from build123d import *

# Parameters (mm, degrees)
SKETCH_1_R               = 4.95
EXTRUDE_1_DEPTH          = 4.5
CUT_EXTRUDE_1_DEPTH      = 2
PATTERN_CIRCULAR_1_COUNT = 6
MIRROR_1_COPY_1_DEPTH    = 2
MIRROR_1_COPY_2_DEPTH    = 2
MIRROR_1_COPY_3_DEPTH    = 2
MIRROR_1_COPY_4_DEPTH    = 2
MIRROR_1_COPY_5_DEPTH    = 2
EXTRUDE_2_DEPTH          = 2.4
SKETCH_5_R               = 4.95
EXTRUDE_3_DEPTH          = 22
CUT_EXTRUDE_2_DEPTH      = 29.583255588
CUT_EXTRUDE_2_DEPTH_BACK = 29.583255588
SKETCH_6_W               = 3
SKETCH_6_H               = 3


with BuildPart() as part:
    # 草图1 → 凸台-拉伸1 (new body)
    with BuildSketch(Plane.XY):
        Circle(SKETCH_1_R)
    extrude_1 = extrude(amount=EXTRUDE_1_DEPTH)

    # 草图2 → 切除-拉伸1 (cut)
    with BuildSketch(Plane(origin=(0, 0, 0), x_dir=(-1, 0, 0), z_dir=(0, 0, -1))):
        with BuildLine():
            Line((0, 4.95), (0, 3.95))
            ThreePointArc((0, 3.95), (1.022335228, 3.815407014), (1.975, 3.420800345))
            Line((1.975, 3.420800345), (2.475, 4.286825749))
            ThreePointArc((2.475, 4.286825749), (1.281154273, 4.78133284), (0, 4.95))
        make_face()
    cut_extrude_1 = extrude(amount=-CUT_EXTRUDE_1_DEPTH, mode=Mode.SUBTRACT)

    # 阵列(圆周)1: 切除-拉伸1 ×6 about axis
    pattern_circular_1_axis = Axis((0, 0, 0), (0, 0, 1))
    for i in range(1, PATTERN_CIRCULAR_1_COUNT):
        add(cut_extrude_1.rotate(pattern_circular_1_axis, i * 360 / PATTERN_CIRCULAR_1_COUNT), mode=Mode.SUBTRACT)

    # 镜向1: 凸台-拉伸1, 切除-拉伸1 across plane
    add(extrude_1.mirror(Plane.XY))
    add(cut_extrude_1.mirror(Plane.XY), mode=Mode.SUBTRACT)

    # 镜向1 copy 1 sketch → 镜向1 copy 1 (cut)
    with BuildSketch(Plane(origin=(0, 0, 0), x_dir=(-0.5000000000000001, -0.8660254037844386, 0), z_dir=(0, 0, 1))):
        with BuildLine():
            Line((0, -4.95), (0, -3.95))
            ThreePointArc((0, -3.95), (1.022335228, -3.815407014), (1.975, -3.420800345))
            Line((1.975, -3.420800345), (2.475, -4.286825749))
            ThreePointArc((2.475, -4.286825749), (1.281154273, -4.78133284), (0, -4.95))
        make_face()
    extrude(amount=-MIRROR_1_COPY_1_DEPTH, mode=Mode.SUBTRACT)

    # 镜向1 copy 2 sketch → 镜向1 copy 2 (cut)
    with BuildSketch(Plane(origin=(0, 0, 0), x_dir=(0.4999999999999998, -0.8660254037844387, 0), z_dir=(0, 0, 1))):
        with BuildLine():
            Line((0, -4.95), (0, -3.95))
            ThreePointArc((0, -3.95), (1.022335228, -3.815407014), (1.975, -3.420800345))
            Line((1.975, -3.420800345), (2.475, -4.286825749))
            ThreePointArc((2.475, -4.286825749), (1.281154273, -4.78133284), (0, -4.95))
        make_face()
    extrude(amount=-MIRROR_1_COPY_2_DEPTH, mode=Mode.SUBTRACT)

    # 镜向1 copy 3 sketch → 镜向1 copy 3 (cut)
    with BuildSketch(Plane.XY):
        with BuildLine():
            Line((0, -4.95), (0, -3.95))
            ThreePointArc((0, -3.95), (1.022335228, -3.815407014), (1.975, -3.420800345))
            Line((1.975, -3.420800345), (2.475, -4.286825749))
            ThreePointArc((2.475, -4.286825749), (1.281154273, -4.78133284), (0, -4.95))
        make_face()
    extrude(amount=-MIRROR_1_COPY_3_DEPTH, mode=Mode.SUBTRACT)

    # 镜向1 copy 4 sketch → 镜向1 copy 4 (cut)
    with BuildSketch(Plane(origin=(0, 0, 0), x_dir=(0.5000000000000004, 0.8660254037844384, 0), z_dir=(0, 0, 1))):
        with BuildLine():
            Line((0, -4.95), (0, -3.95))
            ThreePointArc((0, -3.95), (1.022335228, -3.815407014), (1.975, -3.420800345))
            Line((1.975, -3.420800345), (2.475, -4.286825749))
            ThreePointArc((2.475, -4.286825749), (1.281154273, -4.78133284), (0, -4.95))
        make_face()
    extrude(amount=-MIRROR_1_COPY_4_DEPTH, mode=Mode.SUBTRACT)

    # 镜向1 copy 5 sketch → 镜向1 copy 5 (cut)
    with BuildSketch(Plane(origin=(0, 0, 0), x_dir=(-0.5000000000000001, 0.8660254037844386, 0), z_dir=(0, 0, 1))):
        with BuildLine():
            Line((0, -4.95), (0, -3.95))
            ThreePointArc((0, -3.95), (1.022335228, -3.815407014), (1.975, -3.420800345))
            Line((1.975, -3.420800345), (2.475, -4.286825749))
            ThreePointArc((2.475, -4.286825749), (1.281154273, -4.78133284), (0, -4.95))
        make_face()
    extrude(amount=-MIRROR_1_COPY_5_DEPTH, mode=Mode.SUBTRACT)

    # 草图3 → 凸台-拉伸2 (add)
    with BuildSketch(Plane(origin=(0, 0, -4.5), x_dir=(-1, 0, 0), z_dir=(0, 0, -1))):
        with BuildLine():
            Line((1.75, 7.75), (1.75, -7.75))
            ThreePointArc((1.75, -7.75), (0, -9.5), (-1.75, -7.75))
            Line((-1.75, -7.75), (-1.75, 7.75))
            ThreePointArc((-1.75, 7.75), (0, 9.5), (1.75, 7.75))
        make_face()
    extrude(amount=EXTRUDE_2_DEPTH)

    # 草图5 → 凸台-拉伸3 (add)
    with BuildSketch(Plane.XY.offset(4.5)):
        with Locations(Location((0, 0, 0), (0, 0, 110.703706257))):
            Circle(SKETCH_5_R)
    extrude(amount=EXTRUDE_3_DEPTH)

    # 草图6 → 切除-拉伸2 (cut, two sides: drawn at the far end of the back side and taken through both)
    with BuildSketch(Plane(origin=(0, 0, 0), x_dir=(0, 0, -1), z_dir=(1, 0, 0)).offset(-CUT_EXTRUDE_2_DEPTH_BACK)):
        with Locations((-19, 0)):
            Rectangle(SKETCH_6_W, SKETCH_6_H)
    extrude(amount=CUT_EXTRUDE_2_DEPTH + CUT_EXTRUDE_2_DEPTH_BACK, mode=Mode.SUBTRACT)


solid = part.part
CAD build for the part. Positions are in the model's coordinates, mm. A direction names the side the tool comes from. Coordinates: 2 decimals unless noted, no trailing zeros. Loops run counter-clockwise (first coordinate to the right, second up) from the corner with the lowest first, then second, coordinate; pieces in that order, holes last. Notation, with made-up numbers: (12, 86) -> (53, 86) arc R15 cw to (53, 106) -> close; hole circle Ø6 at (39.5, 76.5). An arc over 180 degrees is marked (long way). One line per item, written item: value.
1. Flat gauge pins, fed straight in: P1, Ø4, axis at y = -5, z = 4, coming from the -X side; P2, Ø1.5, axis at x = 2, z = 22.5, coming from the +Y side; P3, Ø0.5, axis at x = -4.5, z = -1, coming from the +Y side. Where does each tip first touch, or does it go through?
Answers:
P1: stops at x = -3.94
P2: stops at y = 4.79
P3: stops at y = 2.54
2. Slice it at D-D on y = 7.25. Write the cut outline in (x, z).
Answers:
outline: (-1.75, -6.9) -> (1.75, -6.9) -> (1.75, -4.5) -> (-1.75, -4.5) -> close
3. Which spindle directions (+Z, -Z, +X, -X, +Y, -Y) get a long thin tool onto all of the face, cutting with end or side? Do faces 1 (the face through (3, 0, -4.5)), 2 (the face through (3, 3, 2)), 3 (the face through (-1, 4, 2)). Say none if no direction does.
Answers:
face 1: -Z, +X, +Y, -Y
face 2: none
face 3: +Y
4. Slice it at A-A on x = -3. Write the cut outline in (y, z).
Answers:
outline: (-3.94, -4.5) -> (3.94, -4.5) -> (3.94, 26.5) -> (-3.94, 26.5) -> (-3.94, 2) -> (-2.57, 2) -> (-2.57, -2) -> (-3.94, -2) -> close; hole (-1.5, 17.5) -> (1.5, 17.5) -> (1.5, 20.5) -> (-1.5, 20.5) -> close
5. Pull direction Y, two halves, no side cores. Call faces 4 (the face through (0, 7, -4.5)), 5 (the face through (4, -1, 2)), 6 (the face through (0, -9.5, -5.7)): pulls with the +Y half, pulls with the -Y half, needs draft (parallel to the pull), parting line crosses it, or undercut.
Answers:
face 4: needs draft
face 5: undercut
face 6: pulls with the -Y half
6. Drill centre lines: line 1 (Z direction, x = -2, y = -1); line 2 (Z direction, x = -0.25, y = 1); line 3 (Y direction, x = -0.25, z = 19.5). Where is each one in solid material? Low to high. Write a range as [from, to].
Answers:
line 1: z = [-4.5, 17.5], [20.5, 26.5]
line 2: z = [-6.9, 17.5], [20.5, 26.5]
line 3: y = [-4.94, -1.5], [1.5, 4.94]
7. Slice it at B-B on y = 0.75. Write the cut outline in (x, z).
Answers:
outline: (-4.89, -4.5) -> (-1.75, -4.5) -> (-1.75, -6.9) -> (1.75, -6.9) -> (1.75, -4.5) -> (4.89, -4.5) -> (4.89, 17.5) -> (-4.89, 17.5) -> (-4.89, 2) -> (-3.88, 2) -> (-3.88, -2) -> (-4.89, -2) -> close; (-4.89, 20.5) -> (4.89, 20.5) -> (4.89, 26.5) -> (-4.89, 26.5) -> close
8. Slice it at C-C on z = -3.5. Write the cut outline in (x, y).
Answers:
outline: circle Ø9.9 at (0, 0)
